The listing builds one solid part. Answer for the finished solid, in the listing's coordinates (mm). Give positions to 0.01 mm unless a question says otherwise; leave off trailing zeros. Loops run counter-clockwise (first coordinate to the right, second up) from the corner with the lowest first, then second, coordinate; pieces in that order, holes last. Notation, with made-up numbers: M -1.75,15.25 L 37.25,15.25 A4 cw 37.25,20.25 Z; hole C 32.5,31.25 d5. An arc over 180 degrees is marked long. One line per item, written item: value. Start each with the question number.
Q1. The mould has two halves that part along X. Classify faces 1 (the cylindrical face through (123.184, 3.131, -34.029)), 2 (the flat face through (120, 6.35, -13)), 3 (the flat face through (0, 3, -8)): +X half, -X half, draft (parallel to the pull), parting line (faces both ways), or undercut.
Q2. A cutting plane is placed at C-C, the plane z = -22. Determine the outline of the cut face in (x, y).
Q3. Consider L1, parallel to Y at x = 131.3, z = -4.6 (3 decimals); L2, parallel to X at y = 1, z = -36; L3, parallel to Y at x = 50, z = -1. Determine where each line is inside the solid, lowest interval first.
Q4. A cutting plane is placed at A-A, the plane x = 121.2. Determine the outline of the cut face in (y, z).
Q5. A cutting plane is placed at B-B, the plane z = -42. Determine the outline of the cut face in (x, y), and give its area (3 significant figures).
Q6. Flat-ended cylindrical pins translate along their axes: pin 1 (2 mm diameter, centred on x = 30.3, y = 3.175, fed in from -Z); pin 2 (2 mm diameter, centred on x = 182.5, y = 5.5, fed in from -Z); pin 3 (1.5 mm diameter, centred on x = 171.7, y = 3.175, fed in from -Z). Find the tip coordinate at first contact, or state that the pin passes through.
from build123d import *

# Parameters (mm, degrees)
SKETCH1_W                       = 242.4
SKETCH1_H                       = 71.1
BOSS_EXTRUDE1_DEPTH             = 6.35
SKETCH2_OUTSIDE_W               = 294.938
SKETCH2_OUTSIDE_H               = 123.638
CUT_EXTRUDE1_DEPTH              = 10
TAP_DRILL_FOR_M3X0_5_TAP1_D     = 2.5
TAP_DRILL_FOR_M3X0_5_TAP1_DEPTH = 6
TAP_DRILL_FOR_M3X0_5_TAP1_TIP   = 0.751075774
TAP_DRILL_FOR_M6X1_0_TAP1_D     = 5


with BuildPart() as part:
    # Sketch1 → Boss-Extrude1 (new body)
    with BuildSketch(Plane(origin=(0, 0, 0), x_dir=(1, 0, 0), z_dir=(0, 1, 0))):
        with Locations((121.2, 35.55)):
            Rectangle(SKETCH1_W, SKETCH1_H)
    extrude(amount=BOSS_EXTRUDE1_DEPTH)

    # Sketch2 outside → Cut-Extrude1 (cut)
    with BuildSketch(Plane(origin=(0, 6.35, 0), x_dir=(1, 0, 0), z_dir=(0, 1, 0))):
        with Locations((121.2, 35.55)):
            Rectangle(SKETCH2_OUTSIDE_W, SKETCH2_OUTSIDE_H)
        with BuildLine():
            Line((0, 0), (0, 15.796122239))
            Line((0, 15.796122239), (111.2, 35.55))
            ThreePointArc((111.2, 35.55), (121.2, 45.55), (131.2, 35.55))
            Line((131.2, 35.55), (242.4, 15.796122239))
            Line((242.4, 15.796122239), (242.4, 0))
            Line((242.4, 0), (0, 0))
        make_face(mode=Mode.SUBTRACT)
    extrude(amount=-CUT_EXTRUDE1_DEPTH, mode=Mode.SUBTRACT)

    # Tap Drill for M3x0.5 Tap1
    with Locations(Plane.XY):
        with Locations((232.3, 3.175), (10.1, 3.175), (30.3, 3.175), (50.5, 3.175), (70.7, 3.175), (90.9, 3.175), (111.1, 3.175), (131.3, 3.175), (151.5, 3.175), (171.7, 3.175), (191.9, 3.175), (212.1, 3.175)):
            Hole(TAP_DRILL_FOR_M3X0_5_TAP1_D / 2, depth=TAP_DRILL_FOR_M3X0_5_TAP1_DEPTH)
            with Locations((0, 0, -(TAP_DRILL_FOR_M3X0_5_TAP1_DEPTH + TAP_DRILL_FOR_M3X0_5_TAP1_TIP / 2))):  # 118° drill point
                Cone(0, TAP_DRILL_FOR_M3X0_5_TAP1_D / 2, TAP_DRILL_FOR_M3X0_5_TAP1_TIP, mode=Mode.SUBTRACT)

    # Tap Drill for M6x1.0 Tap1 (through all)
    with Locations(Plane(origin=(0, 6.35, 0), x_dir=(1, 0, 0), z_dir=(0, 1, 0))):
        with Locations((121.2, 35.55)):
            Hole(TAP_DRILL_FOR_M6X1_0_TAP1_D / 2)


solid = part.part
Answer block:
1. face 1: undercut
1. face 2: draft
1. face 3: -X half
2. outline: M 34.92,0 L 207.48,0 L 207.48,6.35 L 34.92,6.35 Z
3. L1: 0 to 1.925, 4.425 to 6.35
3. L2: 111.21 to 118.74, 123.66 to 131.19
3. L3: 0 to 2.03, 4.32 to 6.35
4. outline: M 0,-45.55 L 6.35,-45.55 L 6.35,-38.05 L 0,-38.05 Z; M 0,-33.05 L 6.35,-33.05 L 6.35,0 L 0,0 Z
5. outline: M 113.56,0 L 128.84,0 L 128.84,6.35 L 113.56,6.35 Z
5. area: 97.1 mm^2
6. pin 1: z = -21.36
6. pin 2: z = -26.61
6. pin 3: z = -28.49
